```python
from build123d import *

# Parameters (mm, degrees)
SKETCH_1_R          = 10
EXTRUDE_1_DEPTH     = 100
CUT_EXTRUDE_1_DEPTH = 3
CHAMFER_1_SIZE      = 1
CHAMFER_2_SIZE      = 1


with BuildPart() as part:
    # 草图1 → 凸台-拉伸1 (new body)
    with BuildSketch(Plane(origin=(0, 0, 0), x_dir=(0, 0, -1), z_dir=(1, 0, 0))):
        Circle(SKETCH_1_R)
    extrude(amount=EXTRUDE_1_DEPTH)

    # 草图2 → 切除-拉伸1 (cut)
    with BuildSketch(Plane(origin=(0, 10, 0), x_dir=(1, 0, 0), z_dir=(0, 1, 0))):
        with BuildLine():
            Line((13, 3), (27, 3))
            ThreePointArc((27, 3), (30, 0), (27, -3))
            Line((27, -3), (13, -3))
            ThreePointArc((13, -3), (10, 0), (13, 3))
        make_face()
    extrude(amount=-CUT_EXTRUDE_1_DEPTH, mode=Mode.SUBTRACT)

    # 倒角1
    chamfer_1_edges = [part.edges().sort_by_distance(p)[0] for p in [
        (0, 0, 10),
    ]]
    chamfer(chamfer_1_edges, length=CHAMFER_1_SIZE)

    # 倒角2
    chamfer_2_edges = [part.edges().sort_by_distance(p)[0] for p in [
        (100, 0, 10),
    ]]
    chamfer(chamfer_2_edges, length=CHAMFER_2_SIZE)


solid = part.part
```
Work out the finished part from the listing and answer in its coordinate system (mm). A direction names the side the tool comes from. Give positions to 0.01 mm unless a question says otherwise; leave off trailing zeros. Loops run counter-clockwise (first coordinate to the right, second up) from the corner with the lowest first, then second, coordinate; pieces in that order, holes last. Notation, with made-up numbers: (40.5, 20.25) -> (93.5, 20.25) arc R26 ccw to (93.5, 34.25) -> close; hole circle Ø3 at (-4.75, 20). An arc over 180 degrees is marked (long way). Use CSV: the item, a comma, the result in double quotes.
1. The part is cut by section A-A (z = 0). Write down the section's boundary in (x, y), then the cut area to 3 significant figures.
Found:
outline,"(0, -9) -> (1, -10) -> (99, -10) -> (100, -9) -> (100, 9) -> (99, 10) -> (30, 10) -> (30, 7) -> (10, 7) -> (10, 10) -> (1, 10) -> (0, 9) -> close"
area,"1,940 mm^2"
2. The mould has two halves that part along X. Classify faces 1 (the flat face through (100, 0, 0)), 2 (the cylindrical face through (10, 9, 0)), 3 (the flat face through (0, 0, 0)), 4 (the flat face through (20, 7, 0)): +X half, -X half, draft (parallel to the pull), parting line (faces both ways), or undercut.
Found:
face 1,"+X half"
face 2,"undercut"
face 3,"-X half"
face 4,"undercut"
3. Straight lines are drawn through the part: line 1 (Y direction, x = 90.5, z = 0); line 2 (Z direction, x = 54, y = 0.5); line 3 (X direction, y = 8, z = 1). For each, find the intervals that lie inside material, in ascending order.
Found:
line 1,"-10 to 10"
line 2,"-9.99 to 9.99"
line 3,"0 to 10.17, 29.83 to 100"
4. A tool of negligible diameter and unlimited length cuts with its end or side. For faces 5 (the cylindrical face through (30, 9, 0)), 6 (the cylindrical face through (49.31, -9.76, 2.17)), from which of +Z, -Z, +X, -X, +Y, -Y can it reach the whole face along a straight path? Write none if from no direction.
Found:
face 5,"+Y"
face 6,"+X, -X"
5. The part is cut by section B-B (x = 79.5). Write down the section's boundary in (y, z).
Found:
outline,"circle Ø20 at (0, 0)"
6. Flat-ended cylindrical pins translate along their axes: pin 1 Ø3 at (x, z) = (18, -1) entering from +Y; pin 2 Ø2 at (x, y) = (20, 8) entering from -Z; pin 3 Ø4 at (x, z) = (84, 6.5) entering from +Y. Find the tip coordinate at first contact, or state that the pin passes through.
Found:
pin 1,"y = 7"
pin 2,"z = -7.14"
pin 3,"y = 8.93"
